Check sheet for the drawn part. Datum: minimum x, y, z corner. Units: mm. A direction names the side the tool comes from. Give positions to 0.01 mm unless a question says otherwise; leave off trailing zeros. Loops run counter-clockwise (first coordinate to the right, second up) from the corner with the lowest first, then second, coordinate; pieces in that order, holes last. Notation, with made-up numbers: (30.25, 54.5) - (67.25, 54.5) arc R16 cw to (67.25, 70.5) - close; hole circle Ø5 at (-33, 45). An arc over 180 degrees is marked (long way). Use one line per item in the form item = value.
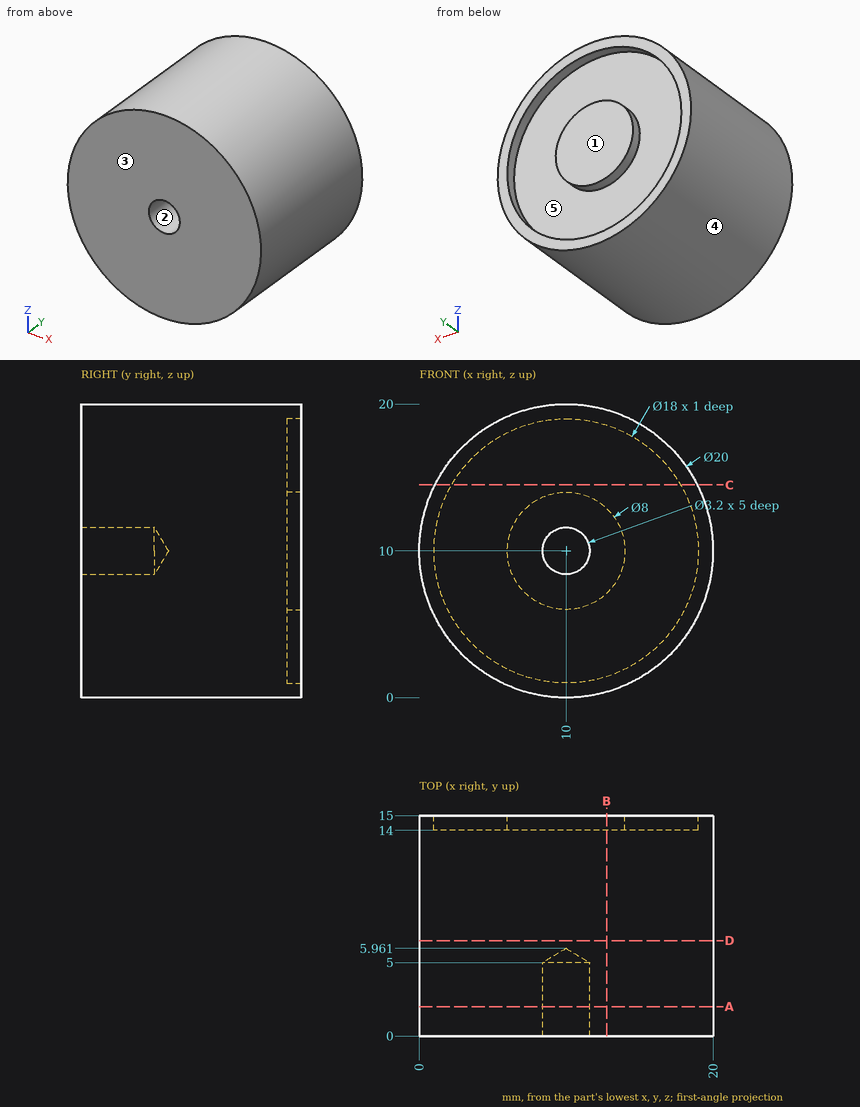
Item 1: Gauge pin test, flat ends, axial feed: P1, Ø2, axis at x = 9, z = 5.5, coming from the -Y side; P2, Ø1, axis at x = 14.5, y = 4, coming from the +Z side (1 decimal); P3, Ø4, axis at x = 15, y = 13, coming from the +Z side; P4, Ø1.5, axis at x = 12, z = 16, coming from the +Y side. Record the tip position at first contact, or that the pin passes through.
Answer block:
P1 = 0
P2 = 19.2
P3 = 19.54
P4 = 14
Item 2: Section check A-A on y = 2. Record the boundary of the cut face in (x, z), then the cut area to 3 significant figures.
Answer block:
outline = circle Ø20 at (10, 10); hole circle Ø3.2 at (10, 10)
area = 306 mm2
Item 3: Mould release check, pull along X, two halves, no side actions. Record for the marked faces 3, 4 and 5: released by +X, released by -X, zero draft, split by the parting line, or undercut.
Answer block:
face_3 = zero draft
face_4 = split by the parting line
face_5 = undercut
Item 4: Section check B-B on x = 12.75. Record the boundary of the cut face in (y, z) (1 decimal), then the cut area to 3 significant figures.
Answer block:
outline = (0, 0.4) - (15, 0.4) - (15, 1.4) - (14, 1.4) - (14, 7.1) - (15, 7.1) - (15, 12.9) - (14, 12.9) - (14, 18.6) - (15, 18.6) - (15, 19.6) - (0, 19.6) - close
area = 277 mm2
Item 5: Thickness scan on L1, parallel to X at y = 14.5, z = 10; L2, parallel to X at y = 3.75, z = 10; L3, parallel to Y at x = 11.25, z = 17.75. Record the ranges inside material, lowest first.
Answer block:
L1 = 0 to 1, 6 to 14, 19 to 20
L2 = 0 to 8.4, 11.6 to 20
L3 = 0 to 14
Item 6: Access from +Z, -Z, +X, -X, +Y, -Y to the whole of each face (thin tool, end or side, straight path). Record for the marked faces 1 and 2.
Answer block:
face_1 = +Z, -Z, +X, -X, +Y
face_2 = -Y
Item 7: Section check C-C on z = 14.5. Record the boundary of the cut face in (x, y).
Answer block:
outline = (1.07, 0) - (18.93, 0) - (18.93, 15) - (17.79, 15) - (17.79, 14) - (2.21, 14) - (2.21, 15) - (1.07, 15) - close
Item 8: Section check D-D on y = 6.5. Record the boundary of the cut face in (x, z), then the cut area to 3 significant figures.
Answer block:
outline = circle Ø20 at (10, 10)
area = 314 mm2
